from build123d import *

# Parameters (mm, degrees)
SKETCH2_R                = 5.15
BOSS_EXTRUDE1_DEPTH      = 3
SKETCH3_R                = 5
SKETCH3_R_2              = 3
BOSS_EXTRUDE2_DEPTH      = 15
BOSS_EXTRUDE2_DEPTH_BACK = 15
SKETCH5_R                = 3
CUT_EXTRUDE1_DEPTH       = 31.0000001


with BuildPart() as part:
    # Sketch2 → Boss-Extrude1 (new body)
    with BuildSketch(Plane.XY):
        with BuildLine():
            Line((4, 0), (10, 0))
            ThreePointArc((10, 0), (12.828427125, 1.171572875), (14, 4))
            Line((14, 4), (14, 16))
            ThreePointArc((14, 16), (12.828427125, 18.828427125), (10, 20))
            Line((10, 20), (4, 20))
            ThreePointArc((4, 20), (1.171572875, 18.828427125), (0, 16))
            Line((0, 16), (0, 4))
            ThreePointArc((0, 4), (1.171572875, 1.171572875), (4, 0))
        make_face()
        with Locations((6.558010351, 6.566011985)):
            Circle(SKETCH2_R, mode=Mode.SUBTRACT)
    extrude(amount=BOSS_EXTRUDE1_DEPTH)

    # Sketch3 → Boss-Extrude2 (add, two sides)
    with BuildSketch(Plane.ZY.offset(-7)) as boss_extrude2_sk:
        with Locations((1.709593121, 19.184703003)):
            Circle(SKETCH3_R)
        with Locations((1.709593121, 19.184703003)):
            Circle(SKETCH3_R_2, mode=Mode.SUBTRACT)
    extrude(amount=BOSS_EXTRUDE2_DEPTH)
    extrude(boss_extrude2_sk.sketch, amount=-BOSS_EXTRUDE2_DEPTH_BACK)

    # Sketch5 → Cut-Extrude1 (cut, through all)
    with BuildSketch(Plane(origin=(22, 0, 0), x_dir=(0, 0, -1), z_dir=(1, 0, 0))):
        with Locations((-1.709593121, 19.184703003)):
            Circle(SKETCH5_R)
    extrude(amount=-CUT_EXTRUDE1_DEPTH, mode=Mode.SUBTRACT)


solid = part.part
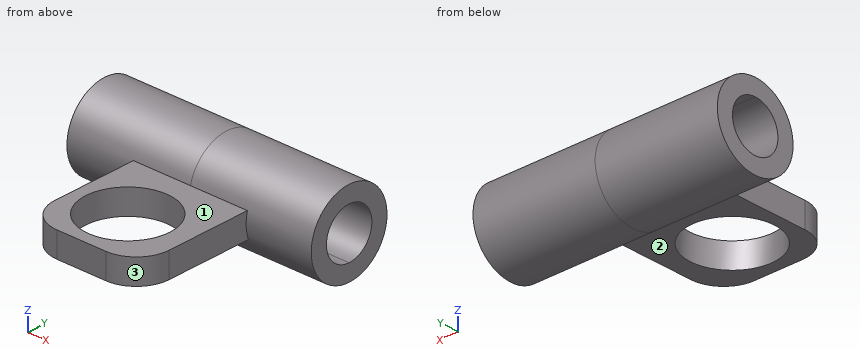
Work out the finished part from the listing and answer in its coordinate system (mm). Face numbers are marked on the shaded views. A direction names the side the tool comes from. Give positions to 0.01 mm unless a question says otherwise; leave off trailing zeros. Loops run counter-clockwise (first coordinate to the right, second up) from the corner with the lowest first, then second, coordinate; pieces in that order, holes last. Notation, with made-up numbers: (46, -34) - (50, -34) arc R24 cw to (50, -23) - close; hole circle Ø10 at (66.25, 66). An arc over 180 degrees is marked (long way). Answer in a Markdown table with one row per item.
(1) Section A-A (x = 4.5) is taken. Give the vertices of the cut face in (y, z).
Results list:
| item | result |
|---|---|
| outline | (0, 0) - (1.85, 0) - (1.85, 3) - (0, 3) - close; (11.29, 0) - (14.49, 0) arc R5 ccw (long way) to (14.35, 3) - (11.29, 3) - close; hole circle Ø6 at (19.18, 1.71) |
(2) Consider L1, parallel to Y at x = -7, z = 1.75; L2, parallel to X at y = 12, z = 2.5; L3, parallel to Y at x = 1, z = 0.25. Determine where each line is inside the solid, lowest interval first. Write a range as [from, to].
Results list:
| item | result |
|---|---|
| L1 | y = [14.18, 16.18], [22.18, 24.18] |
| L2 | x = [0, 14] |
| L3 | y = [1.35, 16.56], [21.81, 23.97] |
(3) Section D-D (z = 4.25) is taken. Give the vertices of the cut face in (x, y), and give its area (3 significant figures).
Results list:
| item | result |
|---|---|
| outline | (-8, 14.88) - (22, 14.88) - (22, 17.59) - (-8, 17.59) - close; (-8, 20.78) - (22, 20.78) - (22, 23.49) - (-8, 23.49) - close |
| area | 163 mm² |
(4) A tool of negligible diameter and unlimited length cuts with its end or side. For the marked faces 1, 2 and 3, from which of +Z, -Z, +X, -X, +Y, -Y can it reach the whole face along a straight path? Write none if from no direction.
Results list:
| item | result |
|---|---|
| face 1 | +Z, +X, -X, -Y |
| face 2 | -Z, +X, -X, -Y |
| face 3 | +Z, -Z, +X, -Y |
(5) Section B-B (z = 0.5) is taken. Give the vertices of the cut face in (x, y), and give its area (3 significant figures).
Results list:
| item | result |
|---|---|
| outline | (-8, 14.33) - (0, 14.33) - (0, 4) arc R4 ccw to (4, 0) - (10, 0) arc R4 ccw to (14, 4) - (14, 14.33) - (22, 14.33) - (22, 16.44) - (-8, 16.44) - close; (-8, 21.93) - (22, 21.93) - (22, 24.04) - (-8, 24.04) - close; hole circle Ø10.3 at (6.56, 6.57) |
| area | 237 mm² |
(6) Flat-ended cylindrical pins translate along their axes: pin 1 Ø5 at (x, z) = (16.5, 5.5) entering from -Y; pin 2 Ø2.5 at (y, z) = (10, 1.5) entering from +X; pin 3 Ø8 at (x, y) = (11.5, 5) entering from +Z; pin 4 Ø1 at (x, y) = (10, 7) entering from +Z. Find the tip coordinate at first contact, or state that the pin passes through.
Results list:
| item | result |
|---|---|
| pin 1 | stops at y = 14.35 |
| pin 2 | stops at x = 14 |
| pin 3 | stops at z = 3 |
| pin 4 | passes through |
(7) Section C-C (y = 18.5) is taken. Give the vertices of the cut face in (x, z).
Results list:
| item | result |
|---|---|
| outline | (-8, -3.24) - (22, -3.24) - (22, -1.21) - (-8, -1.21) - close; (-8, 4.63) - (22, 4.63) - (22, 6.66) - (-8, 6.66) - close |
